```python
from build123d import *

# Parameters (mm, degrees)
F0_W      = 600
F0_H      = 400
F1_DEPTH  = 50
F2_R      = 40
F3_W      = 480
F3_H      = 160
F4_DEPTH  = 49
F5_W      = 480
F5_H      = 10
F6_DEPTH  = 9
F7_T      = -1
F8_W      = 410
F8_H      = 85
F9_DEPTH  = 1.001
F10_W     = 240
F10_H     = 55
F11_DEPTH = 40
F13_DEPTH = 39


with BuildPart() as f1:
    # F0 (on Top) → F1 (new body)
    with BuildSketch(Plane.XY):
        Rectangle(F0_W, F0_H)
    extrude(amount=F1_DEPTH)

    # F2
    f2_edges = [f1.edges().sort_by_distance(p)[0] for p in [
        (0, -200, 50),
        (0, 200, 50),
    ]]
    fillet(f2_edges, radius=F2_R)

    # F3 (on face) → F4 (cut)
    with BuildSketch(Plane.XY.offset(50)):
        Rectangle(F3_W, F3_H)
    extrude(amount=-F4_DEPTH, mode=Mode.SUBTRACT)

    # F5 (on face) → F6 (cut)
    with BuildSketch(Plane.XY.offset(50)):
        with Locations((0, 85)):
            Rectangle(F5_W, F5_H)
        with Locations((0, -85)):
            Rectangle(F5_W, F5_H)
    extrude(amount=-F6_DEPTH, mode=Mode.SUBTRACT)

    # F7
    f7_openings = [f1.faces().sort_by_distance(p)[0] for p in [
        (0, 0, 0),
    ]]
    offset(amount=F7_T, openings=f7_openings, kind=Kind.INTERSECTION)

    # F8 (on face) → F9 (cut, through all)
    with BuildSketch(Plane.XY.offset(1)):
        with Locations((0, -27.5)):
            Rectangle(F8_W, F8_H)
    extrude(amount=-F9_DEPTH, mode=Mode.SUBTRACT)

    # F10 (on face) → F11 (join)
    with BuildSketch(Plane.XY.offset(1)):
        with Locations((-30, 52.5)):
            Rectangle(F10_W, F10_H)
    extrude(amount=F11_DEPTH)

    # F12 (on face) → F13 (join)
    with BuildSketch(Plane.XY.offset(1)):
        with BuildLine():
            Line((-240, -10), (-235, -10))
            ThreePointArc((-235, -10), (-225, 0), (-235, 10))
            Line((-235, 10), (-240, 10))
            Line((-240, 10), (-240, -10))
        make_face()
    extrude(amount=F13_DEPTH)


solid = f1.part
```
Check sheet for the modelled part. Datum: model origin and axes. Units: mm. A direction names the side the tool comes from. Coordinates: 2 decimals unless noted, no trailing zeros. Order: outer loops, then holes, each group sorted by start corner. A loop starts at its lowest first (then second) coordinate and runs counter-clockwise, first axis right, second up. Notation, with made-up numbers: (-8, 66.25) -> (24, 66.25) arc R37 cw to (24, 103.25) -> close; hole circle Ø11 at (78, -21). An arc over 180 degrees is marked (long way). Write each question's results on one line, items separated by ' | '. Start each with the question number.
1) Section check D-D (y = 167.5). Enter the section's corners in (x, z).
2) Set-up check for faces 4 (the face through (164, 80, 21)), 5 (the face through (4.19, 187.88, 37.27)), 6 (the face through (-300, -3, 25)): record each of +Z, -Z, +X, -X, +Y, -Y from which the full face is reachable in a straight line by a thin tool's end or side.
3) Depth check by flat-ended pin: pin 1 (10 mm diameter, centred on x = -230.5, z = 35.5, fed in from +Y); pin 2 (8 mm diameter, centred on x = 128.5, z = 30.5, fed in from +Y); pin 3 (5.5 mm diameter, centred on x = -238.5, z = 19.5, fed in from -Y). Enter the tip coordinate at first touch or a pass-through.
4) Section check B-B (z = 18). Enter the section's corners in (x, y).
5) Material ranges on line 1 along X through (y, z) = (152.5, 8); line 2 along X through (y, z) = (-20.5, 19); line 3 along Y through (x, z) = (198, 10.5), recorded low to high.
6) Draft check along X on faces 1 (the face through (300, -3, 25)), 2 (the face through (-225, 0, 20)), 3 (the face through (4.2, -188.594, 37.972)). Enter one of: pulls with the +X half, pulls with the -X half, needs draft (parallel to the pull), parting line crosses it, or undercut.
7) Section check C-C (y = 0). Enter the section's corners in (x, z).
Checked values:
1) outline: (-300, 0) -> (-299, 0) -> (-299, 48.27) -> (299, 48.27) -> (299, 0) -> (300, 0) -> (300, 49.29) -> (-300, 49.29) -> close
2) face 4: +Z | face 5: -Z | face 6: +Z, -Z, -X, +Y, -Y
3) pin 1: y = 194.35 | pin 2: y = 196.44 | pin 3: y = -199.43
4) outline: (-300, -199.19) -> (300, -199.19) -> (300, 199.19) -> (-300, 199.19) -> close; (-241, -81) -> (241, -81) -> (241, 81) -> (-241, 81) -> close; hole (-299, -198.17) -> (299, -198.17) -> (299, 198.17) -> (-299, 198.17) -> close; hole (-240, -80) -> (240, -80) -> (240, 80) -> (90, 80) -> (90, 25) -> (-150, 25) -> (-150, 80) -> (-240, 80) -> (-240, 10) -> (-235, 10) arc R10 cw to (-235, -10) -> (-240, -10) -> close
5) line 1: -300 to -299, 299 to 300 | line 2: -300 to -299, -241 to -240, 240 to 241, 299 to 300 | line 3: -200 to -199, -81 to -80, 80 to 81, 199 to 200
6) face 1: pulls with the +X half | face 2: undercut | face 3: needs draft
7) outline: (-300, 0) -> (-299, 0) -> (-299, 49) -> (-241, 49) -> (-241, 0) -> (-205, 0) -> (-205, 1) -> (-225, 1) -> (-225, 40) -> (-240, 40) -> (-240, 50) -> (-300, 50) -> close; (205, 0) -> (241, 0) -> (241, 49) -> (299, 49) -> (299, 0) -> (300, 0) -> (300, 50) -> (240, 50) -> (240, 1) -> (205, 1) -> close
